Geometry: final body of the model. Coordinates: model frame, mm. Face numbers are marked on the shaded views. A direction names the side the tool comes from. Give positions to 0.01 mm unless a question says otherwise; leave off trailing zeros. Order: outer loops, then holes, each group sorted by start corner. A loop starts at its lowest first (then second) coordinate and runs counter-clockwise, first axis right, second up. Notation, with made-up numbers: (52, 39) -> (65, 39) arc R29 cw to (65, 60) -> close; hole circle Ø5 at (22.25, 70.5). An arc over 180 degrees is marked (long way). One line per item, written item: value. Start each with the question number.
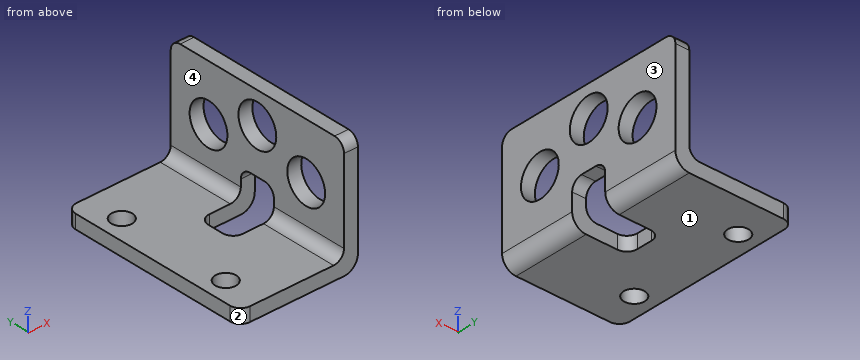
```python
from build123d import *

# Parameters (mm, degrees)
BOSS_EXTRUDE1_DEPTH = 27.5
SKETCH2_R           = 3
CUT_EXTRUDE1_DEPTH  = 27.5
SKETCH3_W           = 6
SKETCH3_H           = 5.25
CUT_EXTRUDE2_DEPTH  = 8
SKETCH4_R           = 1.5
CUT_EXTRUDE3_DEPTH  = 9
FILLET1_R           = 1.5


with BuildPart() as part:
    # Sketch1 → Boss-Extrude1 (new body)
    with BuildSketch(Plane(origin=(0, 0, 0), x_dir=(1, 0, 0), z_dir=(0, 1, 0))):
        with BuildLine():
            Line((0, 0), (15, 0))
            Line((15, 0), (15, -15))
            Line((15, -15), (17, -15))
            Line((17, -15), (17, 0))
            ThreePointArc((17, 0), (16.414213562, 1.414213562), (15, 2))
            Line((15, 2), (0, 2))
            Line((0, 2), (0, 0))
        make_face()
    extrude(amount=BOSS_EXTRUDE1_DEPTH)

    # Sketch2 → Cut-Extrude1 (cut)
    with BuildSketch(Plane(origin=(17, 0, 0), x_dir=(0, 0, -1), z_dir=(1, 0, 0))):
        with Locations((-7, 6)):
            Circle(SKETCH2_R)
        with Locations((-10.5, 13.75)):
            Circle(SKETCH2_R)
        with Locations((-7, 21.5)):
            Circle(SKETCH2_R)
    extrude(amount=-CUT_EXTRUDE1_DEPTH, mode=Mode.SUBTRACT)

    # Sketch3 → Cut-Extrude2 (cut)
    with BuildSketch(Plane(origin=(17, 0, 0), x_dir=(0, 0, -1), z_dir=(1, 0, 0))):
        with Locations((-1, 13.75)):
            Rectangle(SKETCH3_W, SKETCH3_H)
    extrude(amount=-CUT_EXTRUDE2_DEPTH, mode=Mode.SUBTRACT)

    # Sketch4 → Cut-Extrude3 (cut)
    with BuildSketch(Plane(origin=(0, 0, -2), x_dir=(-1, 0, 0), z_dir=(0, 0, -1))):
        with Locations((-3, 5.5)):
            Circle(SKETCH4_R)
        with Locations((-3, 22)):
            Circle(SKETCH4_R)
    extrude(amount=-CUT_EXTRUDE3_DEPTH, mode=Mode.SUBTRACT)

    # Fillet1
    fillet1_edges = [part.edges().sort_by_distance(p)[0] for p in [
        (0, 0, -1),
        (15, 21.9375, 0),
        (16, 27.5, 15),
        (15, 5.5625, 0),
        (16, 11.125, 4),
        (16, 16.375, 4),
        (9, 16.375, -1),
        (9, 11.125, -1),
        (0, 27.5, -1),
        (16, 0, 15),
    ]]
    fillet(fillet1_edges, radius=FILLET1_R)


solid = part.part
```
1. Cut plane A-A, the plane x = 12.75. Return loops of the section in (y, z) (3 decimals), then the cut area to 3 significant figures.
2. Pin query (flat end, axial travel): P1, Ø9.5, axis at y = 6, z = 7, coming from the -X side; P2, Ø2, axis at x = 15.5, y = 14, coming from the -Z side; P3, Ø1.5, axis at x = 4.5, y = 21, coming from the +Z side. Return the tip coordinate at first contact, or that it passes through.
3. Cut plane B-B, the plane y = 15.25. Return loops of the section in (x, z).
4. Access query for the marked faces 3 and 4. Directions: +Z, -Z, +X, -X, +Y, -Y. A direction counts if a zero-diameter tool reaches every point of the face in a straight line with its end or side. Return the directions, or none.
5. Cut plane C-C, the plane x = 3. Return loops of the section in (y, z).
6. Draft query along Y for the marked faces 1 and 2. Return one class per face: pulls with the +Y half, pulls with the -Y half, needs draft (parallel to the pull), parting line crosses it, or undercut.
7. Cut plane D-D, the plane z = 3.5. Return loops of the section in (x, y).
8. Material intervals for L1, parallel to Y at x = 3, z = -1.5; L2, parallel to Y at x = 15.55, z = 7; L3, parallel to Y at x = 16.55, z = 10.5, sorted ascending. Write a range as [from, to].
Answers follow:
1. outline: (0, -2) -> (11.125, -2) -> (11.125, 0) -> (0, 0) -> close; (16.375, -2) -> (27.5, -2) -> (27.5, 0) -> (16.375, 0) -> close
1. area: 44.5 mm²
2. P1: stops at x = 15
2. P2: stops at z = 3.99
2. P3: stops at z = 0
3. outline: (0, -2) -> (9.05, -2) -> (9.05, 0) -> (0, 0) -> close; (15, 3.95) -> (17, 3.95) -> (17, 7.9) -> (15, 7.9) -> close; (15, 13.1) -> (17, 13.1) -> (17, 15) -> (15, 15) -> close
4. face 3: +Z, -Z, +X, +Y, -Y
4. face 4: +Z, -X, +Y, -Y
5. outline: (0, -2) -> (4, -2) -> (4, 0) -> (0, 0) -> close; (7, -2) -> (20.5, -2) -> (20.5, 0) -> (7, 0) -> close; (23.5, -2) -> (27.5, -2) -> (27.5, 0) -> (23.5, 0) -> close
6. face 1: needs draft
6. face 2: pulls with the -Y half
7. outline: (15, 0) -> (17, 0) -> (17, 11.51) -> (15, 11.51) -> close; (15, 15.99) -> (17, 15.99) -> (17, 27.5) -> (15, 27.5) -> close
8. L1: y = [0, 4], [7, 20.5], [23.5, 27.5]
8. L2: y = [0, 3], [9, 18.5], [24.5, 27.5]
8. L3: y = [0, 10.75], [16.75, 27.5]
